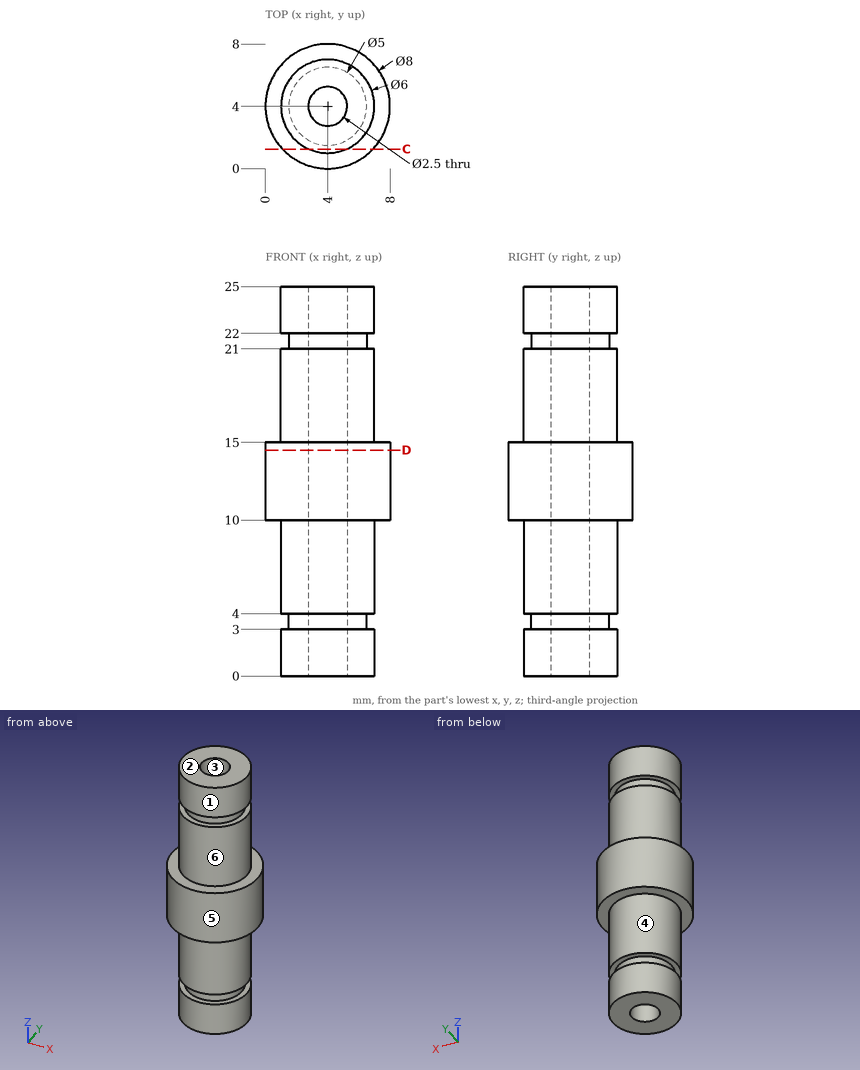
The drawing under review shows one solid part. Ordinate dimensions are in mm from its lowest x, y, z. A direction names the side the tool comes from. Coordinates: 2 decimals unless noted, no trailing zeros. Write each loop counter-clockwise with the first axis right and the second up, starting at its lowest first coordinate (ties: lowest second). Pieces come first, ordered by that corner, then holes. Notation, with made-up numbers: M 29,34 L 43,34 A6 ccw 43,45 Z; hole C 35,55.5 d5. An arc over 180 degrees is marked long. Answer as a JSON object with one key per item and string values.
Item 1: Add section C-C, the plane y = 1.25. Give the boundary of the cut face in (x, z), and give its area (3 significant figures).
Outcome:
{"outline": "M 1.1,10 L 2.8,10 L 2.8,4 L 5.2,4 L 5.2,10 L 6.9,10 L 6.9,15 L 5.2,15 L 5.2,21 L 2.8,21 L 2.8,15 L 1.1,15 Z; M 2.8,0 L 5.2,0 L 5.2,3 L 2.8,3 Z; M 2.8,22 L 5.2,22 L 5.2,25 L 2.8,25 Z", "area": "72.2 mm²"}
Item 2: Machinability: for the marked faces 4, 5 and 6, which of the approach directions +Z, -Z, +X, -X, +Y, -Y give a long, thin tool a straight path to every point of the face, cutting with its end or side? Answer none if there is none.
Outcome:
{"face 4": "-Z", "face 5": "+Z, -Z", "face 6": "+Z"}
Item 3: Wall thickness on probe 1 along Z at (x, y) = (3, 6.5); probe 2 along Y at (x, z) = (4, 9.5); probe 3 along X at (y, z) = (4, 11.75): over which ranges is each line inside the solid? List them lowest first.
Outcome:
{"probe 1": "0 to 3, 4 to 21, 22 to 25", "probe 2": "1 to 2.75, 5.25 to 7", "probe 3": "0 to 2.75, 5.25 to 8"}
Item 4: Draft analysis for pull direction X (two halves, no side actions). For the marked faces 1, 2 and 3, state which applies: pulls with the +X half, pulls with the -X half, needs draft (parallel to the pull), parting line crosses it, or undercut.
Outcome:
{"face 1": "parting line crosses it", "face 2": "needs draft", "face 3": "undercut"}
Item 5: Add section D-D, the plane z = 14.5. Give the boundary of the cut face in (x, y).
Outcome:
{"outline": "C 4,4 d8; hole C 4,4 d2.5"}
Item 6: Insertion check: pin 1 Ø4 at (y, z) = (2.5, 3.5) entering from -X. The pin has a flat end and moves straight along its axis. Give the tip position at first contact, or say it passes through.
Outcome:
{"pin 1": "x = 1"}
